```python
from build123d import *

# Parameters (mm, degrees)
SKETCH1_R           = 6.35
BOSS_EXTRUDE1_DEPTH = 3.175


with BuildPart() as part:
    # Sketch1 → Boss-Extrude1 (new body, symmetric)
    with BuildSketch(Plane.XY):
        Polygon((0, 0), (82.989391896, 0), (19.05, 76.2), (0, 76.2), align=None)
        with Locations((12.7, 63.5)):
            Circle(SKETCH1_R, mode=Mode.SUBTRACT)
        with Locations((12.7, 12.7)):
            Circle(SKETCH1_R, mode=Mode.SUBTRACT)
    extrude(amount=BOSS_EXTRUDE1_DEPTH, both=True)


solid = part.part
```
Part model, mm, in its own coordinate system. Coordinates: 2 decimals unless noted, no trailing zeros. Order: outer loops, then holes, each group sorted by start corner. A loop starts at its lowest first (then second) coordinate and runs counter-clockwise, first axis right, second up. Notation, with made-up numbers: (17, -15) - (72, -15) arc R13 cw to (72, 7) - close; hole circle Ø6 at (12.25, 16). An arc over 180 degrees is marked (long way). Return JSON: item names as keys, results as strings. Group by question number.
Item 1: Pull direction Y, two halves, no side cores. Call faces 1 (the face through (11.32, 57.3, -0.04)), 2 (the face through (0, 39, 0)), 3 (the face through (10, 76.2, 0)): pulls with the +Y half, pulls with the -Y half, needs draft (parallel to the pull), parting line crosses it, or undercut.
Item 2: Cut at A-A (x = 12.7). List the corners of the cut face in (y, z) (3 decimals).
Item 3: Drill centre lines: probe 1 along Y at (x, z) = (12.7, -0.5); probe 2 along Y at (x, z) = (10, -2.75); probe 3 along X at (y, z) = (7, -2.25). Where is each one in solid material? Low to high. Write a range as from..to.
Item 4: Cut at C-C (y = 63.5). List the corners of the cut face in (x, z) (3 decimals), plus the area to 3 significant figures.
Item 5: Cut at B-B (z = -1.5). List the corners of the cut face in (x, y), plus the area to 3 significant figures.
Item 6: Pin check, flat tips, straight feed: pin 1 (2 mm diameter, centred on y = 20, z = -2, fed in from +X); pin 2 (2 mm diameter, centred on y = 55.5, z = 0, fed in from +X). Stop position of each tip, or through.
Item 7: Cut at D-D (y = 12.7). List the corners of the cut face in (x, z) (3 decimals).
Check values:
{
 "1": {"face 1": "undercut", "face 2": "needs draft", "face 3": "pulls with the +Y half"},
 "2": {"outline": "(0, -3.175) - (6.35, -3.175) - (6.35, 3.175) - (0, 3.175) - close; (19.05, -3.175) - (57.15, -3.175) - (57.15, 3.175) - (19.05, 3.175) - close; (69.85, -3.175) - (76.2, -3.175) - (76.2, 3.175) - (69.85, 3.175) - close"},
 "3": {"probe 1": "y = 0..6.35, 19.05..57.15, 69.85..76.2", "probe 2": "y = 0..6.95, 18.45..57.75, 69.25..76.2", "probe 3": "x = 0..9.9, 15.5..77.12"},
 "4": {"outline": "(0, -3.175) - (6.35, -3.175) - (6.35, 3.175) - (0, 3.175) - close; (19.05, -3.175) - (29.707, -3.175) - (29.707, 3.175) - (19.05, 3.175) - close", "area": "108 mm2"},
 "5": {"outline": "(0, 0) - (82.99, 0) - (19.05, 76.2) - (0, 76.2) - close; hole circle Ø12.7 at (12.7, 12.7); hole circle Ø12.7 at (12.7, 63.5)", "area": "3,630 mm2"},
 "6": {"pin 1": "stops at x = 67.05", "pin 2": "stops at x = 37.26"},
 "7": {"outline": "(0, -3.175) - (6.35, -3.175) - (6.35, 3.175) - (0, 3.175) - close; (19.05, -3.175) - (72.333, -3.175) - (72.333, 3.175) - (19.05, 3.175) - close"}
}
